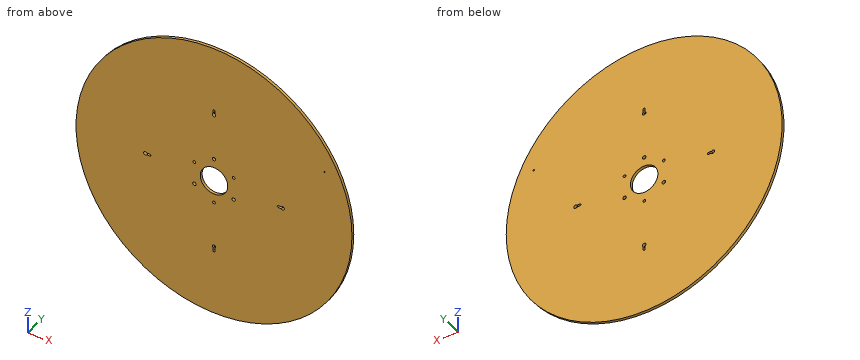
from build123d import *

# Parameters (mm, degrees)
F0_R            = 1004.05
F0_R_2          = 100
F1_DEPTH        = 20
F2_D            = 25
F2_DEPTH        = 28
F2_TIP          = 7.5107577378
F2_COPIES_COUNT = 3
F3_D            = 20
F3_DEPTH        = 28
F3_TIP          = 6.0086061903
F3_COPIES_COUNT = 3
F4_D            = 10
F4_DEPTH        = 28
F4_TIP          = 3.0043030951


# Not quite as in the source:
# - a pattern or mirror of a feature is missing from the dataset's text; its kind, count and spacing are read off the source's solid


with BuildPart() as f1:
    # F0 (on Front) → F1 (new body)
    with BuildSketch(Plane.XZ):
        Circle(F0_R)
        with BuildLine():
            ThreePointArc((12.5, -500), (11.1803398875, -505.5901699437), (7.5, -510))
            Line((7.5, -510), (7.5, -532.5))
            ThreePointArc((7.5, -532.5), (5.3033008589, -537.8033008589), (0, -540))
            ThreePointArc((0, -540), (-5.3033008589, -537.8033008589), (-7.5, -532.5))
            Line((-7.5, -532.5), (-7.5, -510))
            ThreePointArc((-7.5, -510), (-5.5901699437, -488.8196601125), (12.5, -500))
        make_face(mode=Mode.SUBTRACT)
        with BuildLine():
            ThreePointArc((-490, -7.5), (-512.5, 0), (-490, 7.5))
            Line((-490, 7.5), (-467.5, 7.5))
            ThreePointArc((-467.5, 7.5), (-462.1966991411, 5.3033008589), (-460, 0))
            ThreePointArc((-460, 0), (-462.1966991411, -5.3033008589), (-467.5, -7.5))
            Line((-467.5, -7.5), (-490, -7.5))
        make_face(mode=Mode.SUBTRACT)
        Circle(F0_R_2, mode=Mode.SUBTRACT)
        with BuildLine():
            ThreePointArc((512.5, 0), (503.9528470752, -11.8585412256), (490, -7.5))
            Line((490, -7.5), (467.5, -7.5))
            ThreePointArc((467.5, -7.5), (462.1966991411, -5.3033008589), (460, 0))
            ThreePointArc((460, 0), (462.1966991411, 5.3033008589), (467.5, 7.5))
            Line((467.5, 7.5), (490, 7.5))
            ThreePointArc((490, 7.5), (503.9528470752, 11.8585412256), (512.5, 0))
        make_face(mode=Mode.SUBTRACT)
        with BuildLine():
            ThreePointArc((7.5, 510), (11.1803398875, 505.5901699437), (12.5, 500))
            ThreePointArc((12.5, 500), (-5.5901699437, 488.8196601125), (-7.5, 510))
            Line((-7.5, 510), (-7.5, 532.5))
            ThreePointArc((-7.5, 532.5), (-5.3033008589, 537.8033008589), (0, 540))
            ThreePointArc((0, 540), (5.3033008589, 537.8033008589), (7.5, 532.5))
            Line((7.5, 532.5), (7.5, 510))
        make_face(mode=Mode.SUBTRACT)
    extrude(amount=-F1_DEPTH)

    # F2
    with Locations(Plane.XZ):
        with Locations((0, 165)):
            f2 = Hole(F2_D / 2, depth=F2_DEPTH)
            with Locations((0, 0, -(F2_DEPTH + F2_TIP / 2))):  # 118° drill point
                Cone(0, F2_D / 2, F2_TIP, mode=Mode.SUBTRACT)

    # F2_copies: F2 ×3 about axis
    f2_copies_axis = Axis((0, 0, 0), (0, 1, 0))
    for i in range(1, F2_COPIES_COUNT):
        add(f2.rotate(f2_copies_axis, i * 360 / F2_COPIES_COUNT), mode=Mode.SUBTRACT)

    # F3
    with Locations(Plane.XZ):
        with Locations((142.8941916244, 82.5)):
            f3 = Hole(F3_D / 2, depth=F3_DEPTH)
            with Locations((0, 0, -(F3_DEPTH + F3_TIP / 2))):  # 118° drill point
                Cone(0, F3_D / 2, F3_TIP, mode=Mode.SUBTRACT)

    # F3_copies: F3 ×3 about axis
    f3_copies_axis = Axis((0, 0, 0), (0, 1, 0))
    for i in range(1, F3_COPIES_COUNT):
        add(f3.rotate(f3_copies_axis, i * 360 / F3_COPIES_COUNT), mode=Mode.SUBTRACT)

    # F4
    with Locations(Plane.XZ):
        with Locations((804.2584775463, 403.9409626355)):
            Hole(F4_D / 2, depth=F4_DEPTH)
            with Locations((0, 0, -(F4_DEPTH + F4_TIP / 2))):  # 118° drill point
                Cone(0, F4_D / 2, F4_TIP, mode=Mode.SUBTRACT)


solid = f1.part
Geometry: final body of the model. Coordinates: model frame, mm. Round coordinates to 2 decimals unless told otherwise and drop trailing zeros. Loops run counter-clockwise (first coordinate to the right, second up) from the corner with the lowest first, then second, coordinate; pieces in that order, holes last.
Q1. Section A-A on y = 13. State how many separate pieces and enclosed holes the cut face has, plus the area to 3 significant figures.
Q2. Material intervals for L1, parallel to Z at x = 0, y = 4; L2, parallel to X at y = 16.25, z = 5.5; L3, parallel to Z at x = 501.5, y = 10, sorted ascending.
Q3. Pin query (flat end, axial travel): P1, Ø6, axis at x = 579.5, z = 646, coming from the -Y side; P2, Ø4, axis at y = 3.5, z = 454, coming from the +X side; P3, Ø6, axis at y = 11.5, z = 518, coming from the -X side; P4, Ø6, axis at y = 12, z = -521.5, coming from the +X side. Return the tip coordinate at first contact, or that it passes through.
Q4. Section C-C on z = -815.5. Return loops of the section in (x, y).
Q5. Section B-B on x = 387. Return loops of the section in (y, z).
Evaluation:
1. separate pieces: 1
1. enclosed holes: 12
1. area: 3,130,000 mm2
2. L1: z = -1004.05 to -540, -487.5 to -175, -155 to -100, 100 to 152.5, 177.5 to 487.5, 540 to 1004.05
2. L2: x = -1004.03 to -511.22, -462.4 to -99.85, 99.85 to 462.4, 511.22 to 1004.03
2. L3: z = -869.84 to -12.41, 12.41 to 869.84
3. P1: stops at y = 0
3. P2: stops at x = 896.56
3. P3: stops at x = -861.91
3. P4: stops at x = 859.81
4. outline: (-585.73, 0) - (585.73, 0) - (585.73, 20) - (-585.73, 20) - close
5. outline: (0, -926.47) - (20, -926.47) - (20, 926.47) - (0, 926.47) - close
